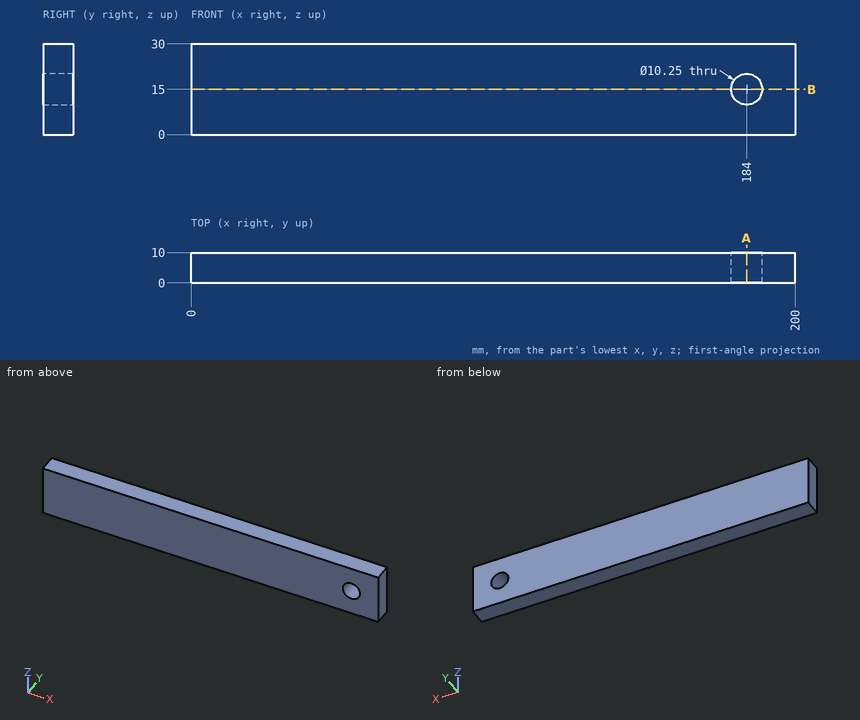
Source: three-view drawing plus pictorial views. Frame: mm from the lowest corner of the part. Coordinates: 2 decimals unless noted, no trailing zeros. Order: outer loops, then holes, each group sorted by start corner. A loop starts at its lowest first (then second) coordinate and runs counter-clockwise, first axis right, second up. Notation, with made-up numbers: M 15,89.5 L 38,89.5 A24 cw 38,120.5 Z; hole C 16.25,17.5 d8. An arc over 180 degrees is marked long. One line per question, with ' | ' between items.
Item 1: Pin query (flat end, axial travel): pin 1 (3 mm diameter, centred on y = 6.5, z = 12.5, fed in from -X). Return the tip coordinate at first contact, or that it passes through.
Geometry results:
pin 1: stops at x = 0
Item 2: Ray query, line 1 along Z through (x, y) = (184, 3.5) (3 decimals); line 2 along X through (y, z) = (4, 15) (3 decimals); line 3 along X through (y, z) = (4, 17.5). Return the intervals inside material, ascending.
Geometry results:
line 1: z = 0 to 9.875, 20.125 to 30 | line 2: x = 0 to 178.875, 189.125 to 200 | line 3: x = 0 to 179.53, 188.47 to 200
Item 3: Section A-A (x = 184). Output: boundary loops of the cut face in (y, z) (3 decimals).
Geometry results:
outline: M 0,0 L 10,0 L 10,9.875 L 0,9.875 Z; M 0,20.125 L 10,20.125 L 10,30 L 0,30 Z
Item 4: Section B-B (z = 15). Output: boundary loops of the cut face in (x, y) (3 decimals).
Geometry results:
outline: M 0,0 L 178.875,0 L 178.875,10 L 0,10 Z; M 189.125,0 L 200,0 L 200,10 L 189.125,10 Z
